Design review of the part built by this model. Coordinates are the model's own, in mm. Face numbers are marked on the shaded views. A direction names the side the tool comes from. Give positions to 0.01 mm unless a question says otherwise; leave off trailing zeros. Loops run counter-clockwise (first coordinate to the right, second up) from the corner with the lowest first, then second, coordinate; pieces in that order, holes last. Notation, with made-up numbers: (73.5, -6) -> (92.5, -6) arc R20 cw to (92.5, 12) -> close; hole circle Ø1 at (21.5, -2). An arc over 180 degrees is marked (long way). Answer in a Markdown table with one row per item. Add a question column.
(1) For line 1 (Y direction, x = -8, z = -45); line 2 (Y direction, x = 39.5, z = 26.5); line 3 (X direction, y = 3.5, z = 0), list the stretches that pass through material, from the lowest coordinate up.
(2) For the marked faces 1 and 2, list the 3-axis set-ups (+Z, -Z, +X, -X, +Y, -Y) from which the entire face can be reached by the end or side of a thin tool; tool diameter is ignored.
(3) Consider section B-B on x = 31.5. Write out the cut boundary in (y, z), then the cut area to 3 significant figures.
(4) Consider section C-C on y = -12.5. Write out the cut boundary in (x, z).
(5) For pin 1 (5 mm diameter, centred on x = 29, z = 13.5, fed in from -Y); pin 2 (2 mm diameter, centred on y = -14, z = 73.5, fed in from +X); pin 3 (5 mm diameter, centred on y = 7, z = 25, fed in from +X), all flat-tipped, find the tip position at first contact; note any pin that passes through.
(6) Consider section A-A on z = 40.5. Write out the cut boundary in (x, y), then the cut area to 3 significant figures.
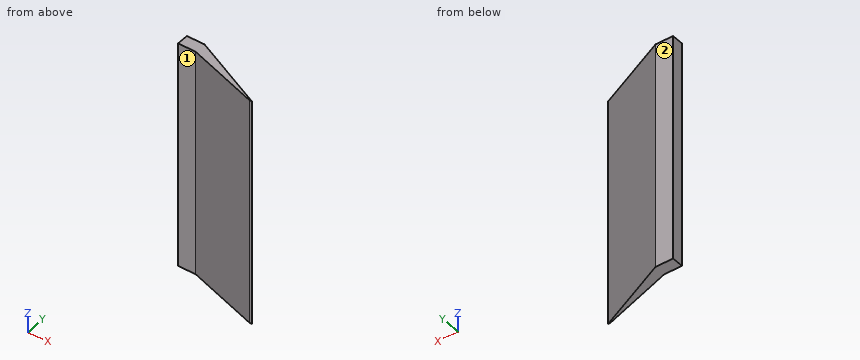
from build123d import *

# Parameters (mm, degrees)
SKETCH3_W           = 195
SKETCH3_H           = 10
BOSS_EXTRUDE1_DEPTH = 15
BOSS_EXTRUDE2_DEPTH = 97.5


with BuildPart() as part:
    # Sketch3 → Boss-Extrude1 (new body)
    with BuildSketch(Plane(origin=(0, 0, 0), x_dir=(0, 0, -1), z_dir=(1, 0, 0))):
        with Locations((0, 5)):
            Rectangle(SKETCH3_W, SKETCH3_H)
    extrude(amount=-BOSS_EXTRUDE1_DEPTH)

    # Sketch4 → Boss-Extrude2 (add, symmetric)
    with BuildSketch(Plane.XY):
        Polygon((61.163603665, -20), (63.163603665, -20), (0, 10), (0, 0), align=None)
    extrude(amount=BOSS_EXTRUDE2_DEPTH, both=True)


solid = part.part
Values follow:
| question | item | result |
|---|---|---|
| 1 | line 1 | 0 to 10 |
| 1 | line 2 | -12.92 to -8.76 |
| 1 | line 3 | -15 to 13.69 |
| 2 | face 1 | +Z, -Z, -X, -Y |
| 2 | face 2 | +Z, -Z, +X, -X, +Y |
| 3 | outline | (-10.3, -97.5) -> (-4.96, -97.5) -> (-4.96, 97.5) -> (-10.3, 97.5) -> close |
| 3 | area | 1,040 mm2 |
| 4 | outline | (38.23, -97.5) -> (47.37, -97.5) -> (47.37, 97.5) -> (38.23, 97.5) -> close |
| 5 | pin 1 | y = -10.3 |
| 5 | pin 2 | x = 52.64 |
| 5 | pin 3 | x = 11.58 |
| 6 | outline | (-15, 0) -> (0, 0) -> (61.16, -20) -> (63.16, -20) -> (0, 10) -> (-15, 10) -> close |
| 6 | area | 486 mm2 |
